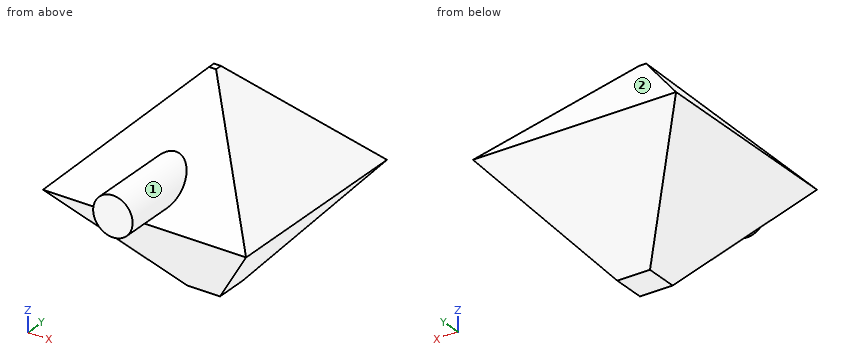
from build123d import *

# Parameters (mm, degrees)
F0_W          = 25.4
F0_H          = 25.4
F1_DEPTH      = 12.7
F1_TAPER      = 44
F1_DEPTH_BACK = 12.7
F1_TAPER_BACK = 40
F4_R          = 2.4668043614
F5_DEPTH      = 14.478


with BuildPart() as f1:
    # F0 (on Top) → F1 (new body, two sides)
    with BuildSketch(Plane.XY) as f1_sk:
        Rectangle(F0_W, F0_H)
    extrude(amount=F1_DEPTH, taper=F1_TAPER)
    extrude(f1_sk.sketch, amount=-F1_DEPTH_BACK, taper=F1_TAPER_BACK)

    # F4 (on face) → F5 (join)
    with BuildSketch(Plane.XZ.offset(3.9232242852)):
        with Locations((0, 3.4155005123)):
            Circle(F4_R)
    extrude(amount=F5_DEPTH)


solid = f1.part
Work out the finished part from the listing and answer in its coordinate system (mm). Face numbers are marked on the shaded views. A direction names the side the tool comes from. Give positions to 0.01 mm unless a question says otherwise; leave off trailing zeros. Loops run counter-clockwise (first coordinate to the right, second up) from the corner with the lowest first, then second, coordinate; pieces in that order, holes last. Notation, with made-up numbers: (68, 44) -> (100, 44) arc R8 ccw to (100, 57) -> close; hole circle Ø11 at (85.25, 44). An arc over 180 degrees is marked (long way). Use a Markdown table: item, result. Add a question column.
1. Find the intervals of material crossed by probe 1 along Y at (x, z) = (0, 9); probe 2 along Z at (x, y) = (-0.5, 3.5); probe 3 along Z at (x, y) = (-0.5, -15), in increasing order.
2. For the marked faces 1 and 2, determine the directions among +Z, -Z, +X, -X, +Y, -Y from which every point of the face is accessible in a straight line to the end or side of a thin tool.
3. Flat-ended cylindrical pins translate along their axes: pin 1 Ø4 at (y, z) = (-6, -7) entering from -X; pin 2 Ø8 at (x, y) = (-9.5, -4.5) entering from -Z; pin 3 Ø3 at (y, z) = (-7, 1) entering from +X; pin 4 Ø1.5 at (x, z) = (5.5, 9) entering from +Y. Find the tip coordinate at first contact, or state that the pin passes through.
4. Section A-A on z = 1.75 is taken. Determine the outline of the cut face in (x, y).
5. Section B-B on z = 10.75 is taken. Determine the outline of the cut face in (x, y), and give its area (3 significant figures).
Results below:
| question | item | result |
|---|---|---|
| 1 | probe 1 | y = -4.01 to 4.01 |
| 1 | probe 2 | z = -10.96 to 9.53 |
| 1 | probe 3 | z = 1 to 5.83 |
| 2 | face 1 | -Y |
| 2 | face 2 | +Z, +X, -X, +Y |
| 3 | pin 1 | stops at x = -8.5 |
| 3 | pin 2 | stops at z = -8.58 |
| 3 | pin 3 | stops at x = 12.7 |
| 3 | pin 4 | passes through |
| 4 | outline | (-11.01, -11.01) -> (-1.82, -11.01) -> (-1.82, -18.4) -> (1.82, -18.4) -> (1.82, -11.01) -> (11.01, -11.01) -> (11.01, 11.01) -> (-11.01, 11.01) -> close |
| 5 | outline | (-2.32, -2.32) -> (2.32, -2.32) -> (2.32, 2.32) -> (-2.32, 2.32) -> close |
| 5 | area | 21.5 mm^2 |
